Geometry check sheet. Reference: the model listing, model coordinates, mm. Give positions to 0.01 mm unless a question says otherwise; leave off trailing zeros. Write each loop counter-clockwise with the first axis right and the second up, starting at its lowest first coordinate (ties: lowest second). Pieces come first, ordered by that corner, then holes. Notation, with made-up numbers: (82, 2.5) -> (134, 2.5) arc R21 ccw to (134, 8.5) -> close; hole circle Ø6 at (74.5, -5). An arc over 180 degrees is marked (long way). Write item = value, one per line. Start each with the question number.
1. Cross-section at A-A, the plane y = -5. Record the cut outline in (x, z), plus the area to 3 significant figures.
2. Cross-section at B-B, the plane x = 0.7. Record the cut outline in (y, z).
3. Depth check by flat-ended pin: P1, Ø2, axis at y = -2.5, z = -1.5, coming from the -X side. Enter the tip coordinate at first touch or a pass-through.
4. Mould release check, pull along Z, two halves, no side actions. Record for faces 1 (the flat face through (0, 0, 0)), 2 (the cylindrical face through (-0.54, -5.92, -2.44)): pulls with the +Z half, pulls with the -Z half, needs draft (parallel to the pull), parting line crosses it, or undercut.
5. Cross-section at C-C, the plane z = 1.65. Record the cut outline in (x, y).
6. Thickness scan on line 1 along Z through (x, y) = (-1.55, -7.25); line 2 along Z through (x, y) = (-1, -3); line 3 along X through (y, z) = (-6, 2.15). Record the ranges inside material, lowest first.
```python
from build123d import *

# Parameters (mm, degrees)
F0_R     = 2.5
F1_DEPTH = 72
F2_DEPTH = 50
F3_DEPTH = 10


with BuildPart() as f1:
    # F0 (on Front) → F1 (new body)
    with BuildSketch(Plane.XZ):
        Circle(F0_R)
    extrude(amount=F1_DEPTH)

    # F2 (cut): a face of the model
    f2_faces = [f1.faces().sort_by_distance(p)[0] for p in [
        (0, -72, 0),
    ]]
    extrude(f2_faces, amount=-F2_DEPTH, mode=Mode.SUBTRACT)

    # F3 (cut): a face of the model
    f3_faces = [f1.faces().sort_by_distance(p)[0] for p in [
        (0, -22, 0),
    ]]
    extrude(f3_faces, amount=-F3_DEPTH, mode=Mode.SUBTRACT)


solid = f1.part
```
Answers:
q1.outline = circle Ø5 at (0, 0)
q1.area = 19.6 mm^2
q2.outline = (-12, -2.4) -> (0, -2.4) -> (0, 2.4) -> (-12, 2.4) -> close
q3.P1 = -2.45
q4.face_1 = needs draft
q4.face_2 = parting line crosses it
q5.outline = (-1.88, -12) -> (1.88, -12) -> (1.88, 0) -> (-1.88, 0) -> close
q6.line_1 = -1.96 to 1.96
q6.line_2 = -2.29 to 2.29
q6.line_3 = -1.28 to 1.28
